The listing builds one solid part. Answer for the finished solid, in the listing's coordinates (mm). A direction names the side the tool comes from. Round coordinates to 2 decimals unless told otherwise and drop trailing zeros. Order: outer loops, then holes, each group sorted by start corner. A loop starts at its lowest first (then second) coordinate and runs counter-clockwise, first axis right, second up. Notation, with made-up numbers: (0.25, 49.25) - (26.25, 49.25) arc R28 cw to (26.25, 85.25) - close; hole circle Ø9 at (59, 32.25). An arc over 180 degrees is marked (long way). One line per item, written item: value. Start each with the question number.
1. For a pull along X with two mould halves and no side action, classify faces 1 (the flat face through (0.1, 3, 4.3)), 2 (the flat face through (3, -3, 3)), 3 (the cylindrical face through (13.67, -1.52, -3.03)), 4 (the cylindrical face through (8.816, 2.958, -16.654)) as released by +X, released by -X, zero draft, split by the parting line, or undercut.
2. A tool of negligible diameter and unlimited length cuts with its end or side. For faces 5 (the flat face through (-4, 0, 14)), 6 (the cylindrical face through (-9.76, 4.48, -2.17)), 7 (the cylindrical face through (18.765, 2.958, 0.806)), from which of +Z, -Z, +X, -X, +Y, -Y can it reach the whole face along a straight path? Write none if from no direction.
3. Section C-C, the plane x = -17.5 is taken. Give the vertices of the cut face in (y, z).
4. Section B-B, the plane y = 4.75 is taken. Give the vertices of the cut face in (x, z).
5. Section D-D, the plane z = 6 is taken. Give the vertices of the cut face in (x, y), then the cut area to 3 significant figures.
6. Flat-ended cylindrical pins translate along their axes: P1, Ø3.5, axis at x = -7, z = 0, coming from the +Y side; P2, Ø1, axis at y = 5, z = 5, coming from the -X side; P3, Ø2, axis at y = 4, z = -13.5, coming from the -X side. Find the tip coordinate at first contact, or state that the pin passes through.
7. Straight lines are drawn through the part: line 1 (X direction, y = 3.9, z = 0); line 2 (X direction, y = -0.7, z = 0); line 3 (X direction, y = 4, z = 14). For each, find the intervals that lie inside material, in ascending order.
from build123d import *

# Parameters (mm, degrees)
SKETCH_1_R      = 21.5
SKETCH_1_R_2    = 4
SKETCH_1_R_3    = 1.5
EXTRUDE_1_DEPTH = 3
SKETCH_2_R      = 21.5
SKETCH_2_R_2    = 1.5
SKETCH_2_R_3    = 10
EXTRUDE_2_DEPTH = 3
EXTRUDE_START   = 3
SKETCH_3_R      = 14
SKETCH_3_R_2    = 1.5
SKETCH_3_R_3    = 4
EXTRUDE_3_DEPTH = 3


with BuildPart() as part:
    # 草图1 → 凸台-拉伸1 (new body)
    with BuildSketch(Plane(origin=(0, 0, 0), x_dir=(1, 0, 0), z_dir=(0, 1, 0))):
        with Locations(Location((0, 0, 0), (0, 0, 270))):
            Circle(SKETCH_1_R)
        with Locations(Location((0, 0, 0), (0, 0, 270))):
            Circle(SKETCH_1_R_2, mode=Mode.SUBTRACT)
        with Locations(Location((0, 7, 0), (0, 0, 270))):
            Circle(SKETCH_1_R_3, mode=Mode.SUBTRACT)
        with Locations(Location((7, 0, 0), (0, 0, 270))):
            Circle(SKETCH_1_R_3, mode=Mode.SUBTRACT)
        with Locations(Location((0, -7, 0), (0, 0, 90))):
            Circle(SKETCH_1_R_3, mode=Mode.SUBTRACT)
        with Locations(Location((-7, 0, 0), (0, 0, 90))):
            Circle(SKETCH_1_R_3, mode=Mode.SUBTRACT)
        with Locations(Location((8.75, 15.155444566, 0), (0, 0, 270))):
            Circle(SKETCH_1_R_3, mode=Mode.SUBTRACT)
        with Locations(Location((17.5, 0, 0), (0, 0, 270))):
            Circle(SKETCH_1_R_3, mode=Mode.SUBTRACT)
        with Locations(Location((-17.5, 0, 0), (0, 0, 90))):
            Circle(SKETCH_1_R_3, mode=Mode.SUBTRACT)
        with Locations(Location((-8.75, 15.155444566, 0), (0, 0, 90))):
            Circle(SKETCH_1_R_3, mode=Mode.SUBTRACT)
        with Locations(Location((8.75, -15.155444566, 0), (0, 0, 90))):
            Circle(SKETCH_1_R_3, mode=Mode.SUBTRACT)
        with Locations(Location((-8.75, -15.155444566, 0), (0, 0, 270))):
            Circle(SKETCH_1_R_3, mode=Mode.SUBTRACT)
    extrude(amount=EXTRUDE_1_DEPTH)

    # 草图2 → 凸台-拉伸2 (add)
    with BuildSketch(Plane(origin=(0, 3, 0), x_dir=(1, 0, 0), z_dir=(0, 1, 0))):
        with Locations(Location((0, 0, 0), (0, 0, 270))):
            Circle(SKETCH_2_R)
        with Locations(Location((-17.5, 0, 0), (0, 0, 90))):
            Circle(SKETCH_2_R_2, mode=Mode.SUBTRACT)
        with Locations(Location((-8.75, -15.155444566, 0), (0, 0, 270))):
            Circle(SKETCH_2_R_2, mode=Mode.SUBTRACT)
        with Locations(Location((8.75, -15.155444566, 0), (0, 0, 90))):
            Circle(SKETCH_2_R_2, mode=Mode.SUBTRACT)
        with Locations(Location((17.5, 0, 0), (0, 0, 270))):
            Circle(SKETCH_2_R_2, mode=Mode.SUBTRACT)
        with Locations(Location((8.75, 15.155444566, 0), (0, 0, 270))):
            Circle(SKETCH_2_R_2, mode=Mode.SUBTRACT)
        with Locations(Location((-8.75, 15.155444566, 0), (0, 0, 90))):
            Circle(SKETCH_2_R_2, mode=Mode.SUBTRACT)
        with Locations(Location((0, 0, 0), (0, 0, 270))):
            Circle(SKETCH_2_R_3, mode=Mode.SUBTRACT)
    extrude(amount=EXTRUDE_2_DEPTH)

    # 草图3 → 凸台-拉伸3 (add)
    with BuildSketch(Plane.XZ.offset(EXTRUDE_START)):
        with Locations(Location((0, 0, 0), (0, 0, 90))):
            Circle(SKETCH_3_R)
        with Locations(Location((7, 0, 0), (0, 0, 270))):
            Circle(SKETCH_3_R_2, mode=Mode.SUBTRACT)
        with Locations(Location((0, 0, 0), (0, 0, 270))):
            Circle(SKETCH_3_R_3, mode=Mode.SUBTRACT)
        with Locations(Location((0, -7, 0), (0, 0, 270))):
            Circle(SKETCH_3_R_2, mode=Mode.SUBTRACT)
        with Locations(Location((-7, 0, 0), (0, 0, 270))):
            Circle(SKETCH_3_R_2, mode=Mode.SUBTRACT)
        with Locations(Location((0, 7, 0), (0, 0, 270))):
            Circle(SKETCH_3_R_2, mode=Mode.SUBTRACT)
    extrude(amount=-EXTRUDE_3_DEPTH)


solid = part.part
Answer list:
1. face 1: undercut
1. face 2: zero draft
1. face 3: split by the parting line
1. face 4: undercut
2. face 5: -Y
2. face 6: +Y
2. face 7: +Y, -Y
3. outline: (0, -12.49) - (6, -12.49) - (6, -1.5) - (0, -1.5) - close; (0, 1.5) - (6, 1.5) - (6, 12.49) - (0, 12.49) - close
4. outline: circle Ø43 at (0, 0); hole circle Ø3 at (-17.5, 0); hole circle Ø3 at (-8.75, -15.16); hole circle Ø3 at (-8.75, 15.16); hole circle Ø20 at (0, 0); hole circle Ø3 at (8.75, -15.16); hole circle Ø3 at (8.75, 15.16); hole circle Ø3 at (17.5, 0)
5. outline: (-20.65, 0) - (-12.65, 0) - (-12.65, -3) - (-1.12, -3) - (-1.12, 3) - (-8, 3) - (-8, 6) - (-20.65, 6) - close; (1.12, -3) - (12.65, -3) - (12.65, 0) - (20.65, 0) - (20.65, 6) - (8, 6) - (8, 3) - (1.12, 3) - close
5. area: 262 mm²
6. P1: stops at y = 3
6. P2: stops at x = -21.02
6. P3: stops at x = -17.49
7. line 1: x = -21.5 to -19, -16 to -10, 10 to 16, 19 to 21.5
7. line 2: x = -14 to -8.5, -5.5 to -4, 4 to 5.5, 8.5 to 14
7. line 3: x = -16.32 to -9.71, -7.79 to 7.79, 9.71 to 16.32
